Design review of the part built by this model. Coordinates are the model's own, in mm. A direction names the side the tool comes from. Give positions to 0.01 mm unless a question says otherwise; leave off trailing zeros. Loops run counter-clockwise (first coordinate to the right, second up) from the corner with the lowest first, then second, coordinate; pieces in that order, holes last. Notation, with made-up numbers: M -17,74 L 37,74 A28 ccw 37,92 Z; hole C 48.5,3 d5. An arc over 180 degrees is marked long. Use a Markdown table: item, result. Add a question column.
(1) Add section A-A, the plane x = 31.75. State how many separate pieces and enclosed holes the cut face has, then the cut area to 3 significant figures.
(2) Draft analysis for pull direction Y (two halves, no side actions). For faces 1 (the face through (33.658, -15.274, 1.565)), 2 (the face through (33.264, 21.114, 1.565)), 3 (the face through (13.494, -8, 8)), 4 (the face through (43.342, 6.641, 1.565)), state which applies: pulls with the +Y half, pulls with the -Y half, needs draft (parallel to the pull), parting line crosses it, or undercut.
(3) Add section D-D, the plane y = 17. Give the boundary of the cut face in (x, z) (1 decimal).
(4) For faces 5 (the face through (36.512, 19, 2)), 6 (the face through (36.512, -15, 2)), 7 (the face through (50.006, -8, 8)), list the 3-axis set-ups (+Z, -Z, +X, -X, +Y, -Y) from which the entire face can be reached by the end or side of a thin tool; tool diameter is ignored.
(5) For probe 1 along Z at (x, y) = (39, 3) (3 decimals); probe 2 along Y at (x, z) = (41, 9.75) (3 decimals); probe 3 along X at (y, z) = (-15.5, 0.75), list the stretches that pass through material, from the lowest coordinate up.
(6) Add section B-B, the plane z = 4.5. Give the boundary of the cut face in (x, y) (3 decimals), then the cut area to 3 significant figures.
(7) Insertion check: pin 1 Ø5 at (x, y) = (31.75, 7.94) entering from +Z (3 decimals); pin 2 Ø2.5 at (y, z) = (17, 1.5) entering from +X; pin 3 Ø3.5 at (y, z) = (-8, 6.5) entering from -X; pin 4 Ø6 at (x, y) = (11.5, -2.5) entering from -Z. Each pin has a flat end and moves straight along its axis. Give the tip position at first contact, or say it passes through.
```python
from build123d import *

# Parameters (mm, degrees)
F0_R     = 2
F0_R_2   = 1.5875
F1_DEPTH = 3.175
F2_W     = 9.525
F2_H     = 3.175
F3_DEPTH = 9.525
F4_R     = 2
F5_DEPTH = 34.926


# Not quite as in the source:
# - a length typed as a fraction of an inch, garbled in the dataset ("3 / 203.2 mm" for 3/8 in), is restored
# - a pattern or mirror of a feature is missing from the dataset's text; its kind, count and spacing are read off the source's solid


with BuildPart() as f1:
    # F0 (on Top) → F1 (new body)
    with BuildSketch(Plane.XY):
        Polygon((13.5171158184, 0), (0, 0), (0, -9.525), (26.9875, -9.525), (26.9875, -20.6375), (36.5125, -20.6375), (36.5125, -9.525), (63.5, -9.525), (63.5, 0), (49.9828841816, 0), (36.5125, 13.4703841816), (36.5125, 25.4), (26.9875, 25.4), (26.9875, 13.4703841816), align=None)
        with Locations((4.7625, -4.7625)):
            Circle(F0_R, mode=Mode.SUBTRACT)
        with Locations((31.75, -15.875)):
            Circle(F0_R, mode=Mode.SUBTRACT)
        with Locations((58.7375, -4.7625)):
            Circle(F0_R, mode=Mode.SUBTRACT)
        with Locations((31.75, 7.9375)):
            Circle(F0_R_2, mode=Mode.SUBTRACT)
        with Locations((31.75, 20.6375)):
            Circle(F0_R_2, mode=Mode.SUBTRACT)
    extrude(amount=F1_DEPTH)

    # F2 (on face) → F3 (join)
    with BuildSketch(Plane.XY.offset(3.175)):
        with Locations((18.25625, -7.9375)):
            Rectangle(F2_W, F2_H)
        with Locations((45.24375, -7.9375)):
            Rectangle(F2_W, F2_H)
    extrude(amount=F3_DEPTH)

    # F4 (on face) → F5 (cut, through all)
    with BuildSketch(Plane.XZ.offset(9.525)):
        with Locations((18.25625, 7.9375)):
            Circle(F4_R)
    f5 = extrude(amount=-F5_DEPTH, mode=Mode.SUBTRACT)

    # F5_copies: F5 across plane
    add(f5.mirror(Plane(origin=(31.75, 0, 0), x_dir=(0, 0, 1), z_dir=(1, 0, 0))), mode=Mode.SUBTRACT)


solid = f1.part
```
Established:
| question | item | result |
|---|---|---|
| 1 | separate pieces | 4 |
| 1 | enclosed holes | 0 |
| 1 | area | 113 mm^2 |
| 2 | face 1 | undercut |
| 2 | face 2 | undercut |
| 2 | face 3 | needs draft |
| 2 | face 4 | pulls with the +Y half |
| 3 | outline | M 27,0 L 36.5,0 L 36.5,3.2 L 27,3.2 Z |
| 4 | face 5 | +Z, -Z, +X, +Y |
| 4 | face 6 | +Z, -Z, +X, -Y |
| 4 | face 7 | +Z, +X, +Y, -Y |
| 5 | probe 1 | 0 to 3.175 |
| 5 | probe 2 | -9.525 to -6.35 |
| 5 | probe 3 | 26.99 to 29.79, 33.71 to 36.51 |
| 6 | outline | M 13.494,-9.525 L 23.019,-9.525 L 23.019,-6.35 L 13.494,-6.35 Z; M 40.481,-9.525 L 50.006,-9.525 L 50.006,-6.35 L 40.481,-6.35 Z |
| 6 | area | 60.5 mm^2 |
| 7 | pin 1 | z = 3.175 |
| 7 | pin 2 | x = 36.51 |
| 7 | pin 3 | x = 13.49 |
| 7 | pin 4 | z = 0 |
